from build123d import *

# Parameters (mm, degrees)
SKETCH1_R           = 1.5
BOSS_EXTRUDE1_DEPTH = 3
SKETCH2_W           = 35
SKETCH2_H           = 3
BOSS_EXTRUDE2_DEPTH = 60


with BuildPart() as part:
    # Sketch1 → Boss-Extrude1 (new body)
    with BuildSketch(Plane.XY):
        with BuildLine():
            Line((-17.5, 0), (-17.5, -20))
            Line((-17.5, -20), (17.5, -20))
            Line((17.5, -20), (17.5, 0))
            ThreePointArc((17.5, 0), (0, 17.5), (-17.5, 0))
        make_face()
        with Locations((0, 14)):
            Circle(SKETCH1_R, mode=Mode.SUBTRACT)
        with Locations((14, 0)):
            Circle(SKETCH1_R, mode=Mode.SUBTRACT)
        with Locations((0, -14)):
            Circle(SKETCH1_R, mode=Mode.SUBTRACT)
        with Locations((-14, 0)):
            Circle(SKETCH1_R, mode=Mode.SUBTRACT)
    extrude(amount=BOSS_EXTRUDE1_DEPTH)

    # Sketch2 → Boss-Extrude2 (add)
    with BuildSketch(Plane(origin=(0, 0, 0), x_dir=(-1, 0, 0), z_dir=(0, 0, -1))):
        with Locations((0, -18.5)):
            Rectangle(SKETCH2_W, SKETCH2_H)
    extrude(amount=BOSS_EXTRUDE2_DEPTH)


solid = part.part
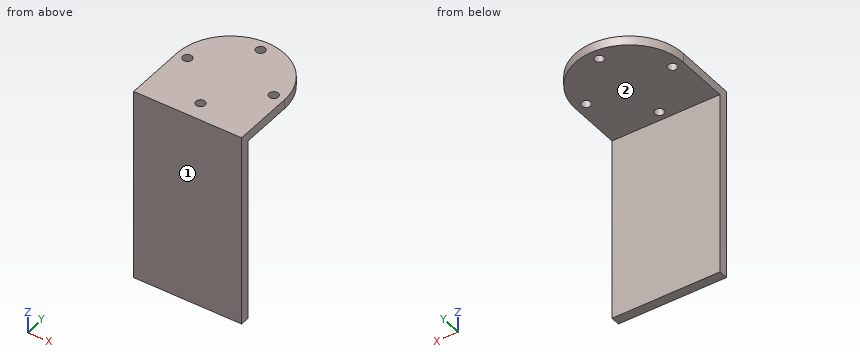
Could you check a few things on this model? Use its own coordinates, in mm. Face numbers are marked on the shaded views. A direction names the side the tool comes from. Coordinates: 2 decimals unless noted, no trailing zeros. Write each loop counter-clockwise with the first axis right and the second up, starting at its lowest first coordinate (ties: lowest second). Pieces come first, ordered by that corner, then holes. Notation, with made-up numbers: M -12.75,26.25 L 21.25,26.25 A15 ccw 21.25,33.25 Z; hole C 16,-1 d6. An arc over 180 degrees is marked long. One line per question, with ' | ' between items.
1) Imagine slicing it at C-C, the plane x = 0. Write out the boundary of the cut face in (y, z), and give its area (4 significant figures).
Checks:
outline: M -20,-60 L -17,-60 L -17,0 L -15.5,0 L -15.5,3 L -20,3 Z; M -12.5,0 L 12.5,0 L 12.5,3 L -12.5,3 Z; M 15.5,0 L 17.5,0 L 17.5,3 L 15.5,3 Z | area: 274.5 mm²
2) Imagine slicing it at B-B, the plane x = -14. Write out the boundary of the cut face in (y, z), and give its area (4 significant figures).
Checks:
outline: M -20,-60 L -17,-60 L -17,0 L -1.5,0 L -1.5,3 L -20,3 Z; M 1.5,0 L 10.5,0 L 10.5,3 L 1.5,3 Z | area: 262.5 mm²
3) Imagine slicing it at A-A, the plane y = 14. Write out the boundary of the cut face in (x, z), and give its area (3 significant figures).
Checks:
outline: M -10.5,0 L -1.5,0 L -1.5,3 L -10.5,3 Z; M 1.5,0 L 10.5,0 L 10.5,3 L 1.5,3 Z | area: 54.0 mm²
4) I need wall thicknesses on probe 1 along Y at (x, z) = (0, 1); probe 2 along Z at (x, y) = (4.5, -13); probe 3 along Y at (x, z) = (12, -13.5). Which ranges of each line are inside material? Lowest first, please. Write a range as [from, to].
Checks:
probe 1: [-20, -15.5], [-12.5, 12.5], [15.5, 17.5] | probe 2: [0, 3] | probe 3: [-20, -17]
5) For the marked faces 1 and 2, which set-ups out of +Z, -Z, +X, -X, +Y, -Y let a thin tool reach every point of the face, with its end or its side?
Checks:
face 1: +Z, -Z, +X, -X, -Y | face 2: -Z, +X, -X, +Y
6) Imagine slicing it at D-D, the plane y = -8. Write out the boundary of the cut face in (x, z), and give its area (3 significant figures).
Checks:
outline: M -17.5,0 L 17.5,0 L 17.5,3 L -17.5,3 Z | area: 105 mm²
7) For pin 1 Ø8 at (x, z) = (-2.5, -49.5) entering from +Y; pin 2 Ø3.5 at (x, y) = (14, 0) entering from -Z, each with a flat end and sliding along its axis, tell me the tip position at first contact or that it passes through.
Checks:
pin 1: y = -17 | pin 2: z = 0
